Source: three-view drawing plus pictorial views. Frame: mm from the lowest corner of the part. A direction names the side the tool comes from. Give positions to 0.01 mm unless a question says otherwise; leave off trailing zeros. Order: outer loops, then holes, each group sorted by start corner. A loop starts at its lowest first (then second) coordinate and runs counter-clockwise, first axis right, second up. Notation, with made-up numbers: (-18.5, -34) -> (-6.5, -34) arc R16 ccw to (-6.5, -8) -> close; hole circle Ø2 at (59.5, 11). An arc over 180 degrees is marked (long way). Answer in a Markdown table with one row per item. Add a question column.
Q1. Cut plane D-D on x = 23.5. Return the cut outline in (y, z), and give its area (3 significant figures).
Q2. Cut plane A-A on y = 30. Return the cut outline in (x, z).
Q3. Set-up query: the marked faces 4, 5 and 6. Return all of +Z, -Z, +X, -X, +Y, -Y with unobstructed straight access to the full face (end or side cutting, diameter ignored); none if empty.
Q4. Line query: line 1 along Y through (x, z) = (30, 1.5); line 2 along Z through (x, y) = (11, 29); line 3 along Y through (x, z) = (11, 5) (1 decimal). Output: solid intervals per line, ascending. Write a range as from..to.
Q5. Pull-direction query (Y, two-part tool) for the marked faces 1, 2 and 3; classes: +Y half, -Y half, draft (parallel to the pull), parting line (faces both ways), or undercut.
Q6. Cut plane B-B on z = 7. Return the cut outline in (x, y), and give its area (3 significant figures).
Q7. Cut plane C-C on y = 18.75. Return the cut outline in (x, z) (1 decimal).
Q8. Contact query for flat-ended pins moving along their axis: P1, Ø2, axis at y = 30, z = 24, coming from the +X side; P2, Ø7, axis at x = 10.51, y = 18.75, coming from the +Z side; P3, Ø12, axis at y = 19, z = 35, coming from the -X side. Output: stop coordinate, or through.
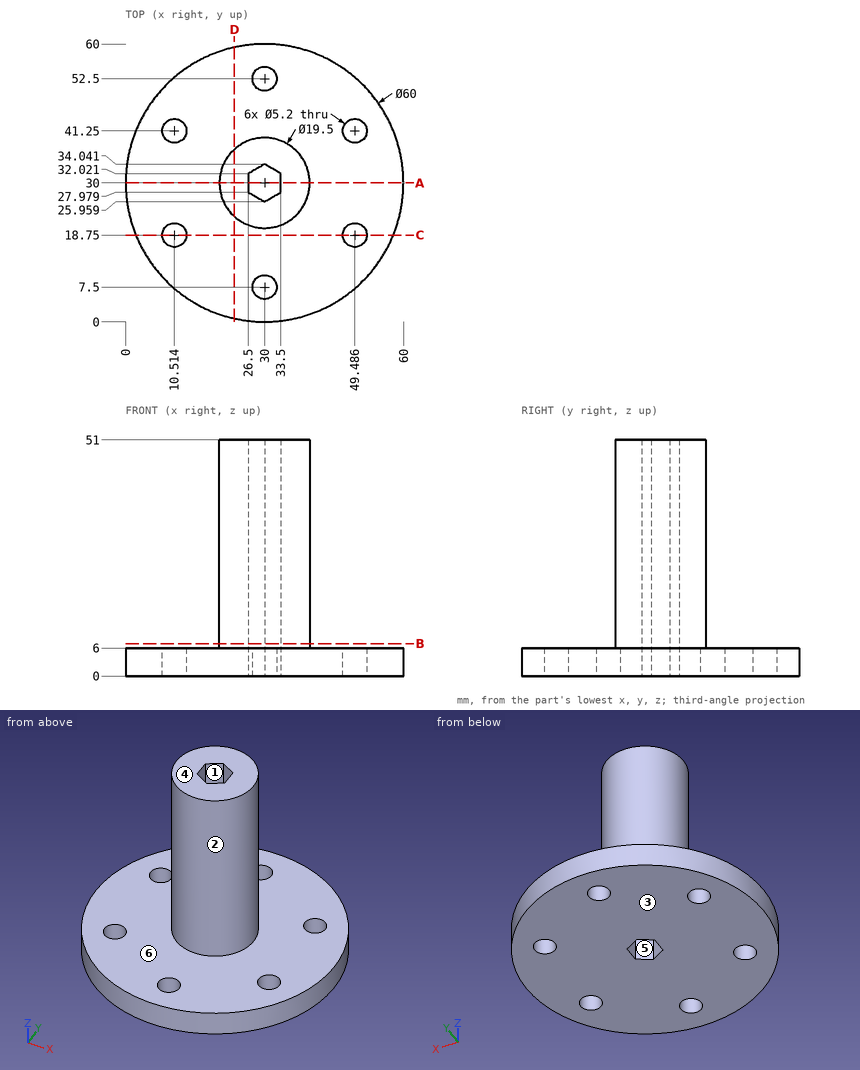
Completed:
| question | item | result |
|---|---|---|
| 1 | outline | (0.71, 0) -> (59.29, 0) -> (59.29, 6) -> (37.27, 6) -> (37.27, 51) -> (22.73, 51) -> (22.73, 6) -> (0.71, 6) -> close |
| 1 | area | 1,010 mm² |
| 2 | outline | (0, 0) -> (26.5, 0) -> (26.5, 51) -> (20.25, 51) -> (20.25, 6) -> (0, 6) -> close; (33.5, 0) -> (60, 0) -> (60, 6) -> (39.75, 6) -> (39.75, 51) -> (33.5, 51) -> close |
| 3 | face 4 | +Z, +X, -X, +Y, -Y |
| 3 | face 5 | +Z, -Z |
| 3 | face 6 | +Z |
| 4 | line 1 | y = 0..4.9, 10.1..25.96, 34.04..49.9, 55.1..60 |
| 4 | line 2 | z = 0..6 |
| 4 | line 3 | y = 6.8..16.2, 21.3..38.7, 43.8..53.2 |
| 5 | face 1 | undercut |
| 5 | face 2 | parting line |
| 5 | face 3 | draft |
| 6 | outline | circle Ø19.5 at (30, 30); hole (26.5, 27.98) -> (30, 25.96) -> (33.5, 27.98) -> (33.5, 32.02) -> (30, 34.04) -> (26.5, 32.02) -> close |
| 6 | area | 256 mm² |
| 7 | outline | (2.2, 0) -> (7.9, 0) -> (7.9, 6) -> (2.2, 6) -> close; (13.1, 0) -> (46.9, 0) -> (46.9, 6) -> (13.1, 6) -> close; (52.1, 0) -> (57.8, 0) -> (57.8, 6) -> (52.1, 6) -> close |
| 8 | P1 | stops at x = 39.75 |
| 8 | P2 | stops at z = 6 |
| 8 | P3 | stops at x = 21.63 |
